Design review of the part built by this model. Coordinates are the model's own, in mm. Face numbers are marked on the shaded views. A direction names the side the tool comes from. Round coordinates to 2 decimals unless told otherwise and drop trailing zeros. Loops run counter-clockwise (first coordinate to the right, second up) from the corner with the lowest first, then second, coordinate; pieces in that order, holes last. Notation, with made-up numbers: (55, -4) - (106, -4) arc R29 cw to (106, 27) - close; hole circle Ø10 at (53, -17.5). An arc over 180 degrees is marked (long way). Use one line per item in the form item = value. Start each with the question number.
(1) We need section D-D, the plane x = 23.5. Write out the cut boundary in (y, z).
(2) For pin 1 (6 mm diameter, centred on x = 30.5, z = 15.5, fed in from -Y); pin 2 (3 mm diameter, centred on y = 4.5, z = 1.5, fed in from -X); pin 3 (3 mm diameter, centred on x = 52.5, z = 10.5, fed in from +Y), all flat-tipped, find the tip position at first contact; note any pin that passes through.
(3) Wall thickness on probe 1 along Z at (x, y) = (0, 3.5); probe 2 along Z at (x, y) = (31.95, -2.15); probe 3 along X at (y, z) = (5.1, 13.8): over which ranges is each line inside the solid? List them lowest first. Write a range as [from, to].
(4) The part is to be moulded in two halves that separate along Z. For the marked faces 1, 2, 3 and 4, say which applies: released by +Z, released by -Z, zero draft, split by the parting line, or undercut.
(5) We need section C-C, the plane z = -13.8. Write out the cut boundary in (x, y), then the cut area to 3 significant figures.
(6) We need section A-A, the plane x = 7.5. Write out the cut boundary in (y, z).
(7) Machinability: for the marked faces 5, 6, 7 and 8, which of the approach directions +Z, -Z, +X, -X, +Y, -Y give a long, thin tool a straight path to every point of the face, cutting with its end or side? Answer none if there is none.
(8) We need section B-B, the plane x = 55.95. Write out the cut boundary in (y, z).
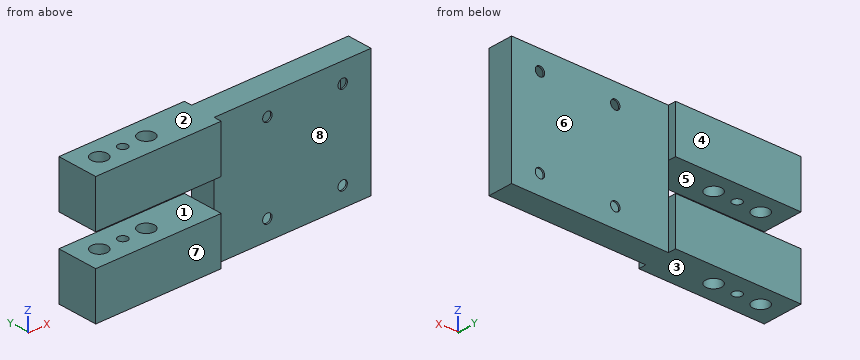
from build123d import *

# Parameters (mm, degrees)
BOSS_EXTRUDE1_DEPTH             = 5
BOSS_EXTRUDE1_DEPTH_BACK        = 5
SHELL1_T                        = -3
BOSS_EXTRUDE2_START             = 5
BOSS_EXTRUDE2_DEPTH             = 3
SKETCH2_R                       = 1.5
CUT_EXTRUDE1_DEPTH              = 100
SKETCH9_W                       = 40
SKETCH9_H                       = 2.5
CUT_EXTRUDE2_DEPTH              = 77.739820172
SKETCH10_W                      = 10
SKETCH10_H                      = 40
CUT_EXTRUDE3_DEPTH              = 2.5
CUT_EXTRUDE4_START              = -10.5
SKETCH10_2_W                    = 10
SKETCH10_2_H                    = 40
CUT_EXTRUDE4_DEPTH              = 2.5
F_3_0MM_CLEARANCE_DOWEL_HOLE1_D = 3
F_1_4_20_TAPPED_HOLE1_D         = 5.1054


with BuildPart() as part:
    # Sketch1 → Boss-Extrude1 (new, two sides: drawn at the far end of the back side and taken through both)
    with BuildSketch(Plane(origin=(0, 0, 0), x_dir=(1, 0, 0), z_dir=(0, 1, 0)).offset(-BOSS_EXTRUDE1_DEPTH_BACK)):
        Polygon((15, -5), (-25, -5), (-25, -20), (25, -20), (65, -20), (65, 20), (25, 20), (-25, 20), (-25, 5), (15, 5), align=None)
    extrude(amount=BOSS_EXTRUDE1_DEPTH + BOSS_EXTRUDE1_DEPTH_BACK)

    # Shell1
    shell1_openings = [part.faces().sort_by_distance(p)[0] for p in [
        (23.125, 5, 0),
    ]]
    offset(amount=SHELL1_T, openings=shell1_openings, kind=Kind.INTERSECTION)

    # Sketch1<2> → Boss-Extrude2 (add)
    with BuildSketch(Plane(origin=(0, 0, 0), x_dir=(1, 0, 0), z_dir=(0, 1, 0)).offset(BOSS_EXTRUDE2_START)):
        Polygon((15, -5), (-25, -5), (-25, -20), (25, -20), (65, -20), (65, 20), (25, 20), (-25, 20), (-25, 5), (15, 5), align=None)
    extrude(amount=BOSS_EXTRUDE2_DEPTH)

    # Sketch2 → Cut-Extrude1 (cut)
    with BuildSketch(Plane.XY.offset(20)):
        with Locations((-10.5, 1.5)):
            Circle(SKETCH2_R)
    extrude(amount=-CUT_EXTRUDE1_DEPTH, mode=Mode.SUBTRACT)

    # Sketch9 → Cut-Extrude2 (cut, through all)
    with BuildSketch(Plane.XY.offset(20)):
        with Locations((45, 6.75)):
            Rectangle(SKETCH9_W, SKETCH9_H)
        with Locations((45, -3.75)):
            Rectangle(SKETCH9_W, SKETCH9_H)
    extrude(amount=-CUT_EXTRUDE2_DEPTH, mode=Mode.SUBTRACT)

    # Sketch10 → Cut-Extrude3 (cut)
    with BuildSketch(Plane(origin=(0, 8, 0), x_dir=(1, 0, 0), z_dir=(0, 1, 0))):
        with Locations((20, 0)):
            Rectangle(SKETCH10_W, SKETCH10_H)
    extrude(amount=-CUT_EXTRUDE3_DEPTH, mode=Mode.SUBTRACT)

    # Sketch10<2> → Cut-Extrude4 (cut)
    with BuildSketch(Plane(origin=(0, 8, 0), x_dir=(1, 0, 0), z_dir=(0, 1, 0)).offset(CUT_EXTRUDE4_START)):
        with Locations((20, 0)):
            Rectangle(SKETCH10_2_W, SKETCH10_2_H)
    extrude(amount=-CUT_EXTRUDE4_DEPTH, mode=Mode.SUBTRACT)

    # Ø3.0mm Clearance Dowel Hole1 (through all)
    with Locations(Plane(origin=(0, 5.5, 0), x_dir=(1, 0, 0), z_dir=(0, 1, 0))):
        with Locations((31.950000364, 13.8), (31.950000364, -13.8), (55.950000364, -13.8), (55.950000364, 13.8)):
            Hole(F_3_0MM_CLEARANCE_DOWEL_HOLE1_D / 2)

    # 1/4-20 Tapped Hole1 (through all)
    with Locations(Plane.XY.offset(20)):
        with Locations((-18, 1.5), (-3, 1.5)):
            Hole(F_1_4_20_TAPPED_HOLE1_D / 2)


solid = part.part
Data:
q1.outline = (-2.5, -20) - (5.5, -20) - (5.5, 20) - (-2.5, 20) - close; hole (-2, -17) - (5, -17) - (5, 17) - (-2, 17) - close
q2.pin_1 = -2.5
q2.pin_2 = 15
q2.pin_3 = 5.5
q3.probe_1 = [-20, -17], [-8, -5], [5, 8], [17, 20]
q3.probe_2 = [-20, -15.3], [-12.3, 12.3], [15.3, 20]
q3.probe_3 = [-25, 30.45], [33.45, 54.45], [57.45, 65]
q4.face_1 = undercut
q4.face_2 = released by +Z
q4.face_3 = released by -Z
q4.face_4 = zero draft
q5.outline = (-25, -5) - (15, -5) - (15, -2.5) - (30.45, -2.5) - (30.45, -2) - (-22, -2) - (-22, 5) - (30.45, 5) - (30.45, 5.5) - (15, 5.5) - (15, 8) - (-25, 8) - close; (33.45, -2.5) - (54.45, -2.5) - (54.45, -2) - (33.45, -2) - close; (33.45, 5) - (54.45, 5) - (54.45, 5.5) - (33.45, 5.5) - close; (57.45, -2.5) - (65, -2.5) - (65, 5.5) - (57.45, 5.5) - (57.45, 5) - (62, 5) - (62, -2) - (57.45, -2) - close
q5.area = 326 mm^2
q6.outline = (-5, -20) - (8, -20) - (8, -5) - (-5, -5) - close; (-5, 5) - (8, 5) - (8, 20) - (-5, 20) - close; hole (-2, -17) - (5, -17) - (5, -8) - (-2, -8) - close; hole (-2, 8) - (5, 8) - (5, 17) - (-2, 17) - close
q7.face_5 = -X, +Y, -Y
q7.face_6 = +Z, -Z, +X, +Y
q7.face_7 = +Z, -Z, +X, -X, -Y
q7.face_8 = +Z, -Z, +X, -Y
q8.outline = (-2.5, -20) - (5.5, -20) - (5.5, -15.3) - (5, -15.3) - (5, -17) - (-2, -17) - (-2, -15.3) - (-2.5, -15.3) - close; (-2.5, -12.3) - (-2, -12.3) - (-2, 12.3) - (-2.5, 12.3) - close; (-2.5, 15.3) - (-2, 15.3) - (-2, 17) - (5, 17) - (5, 15.3) - (5.5, 15.3) - (5.5, 20) - (-2.5, 20) - close; (5, -12.3) - (5.5, -12.3) - (5.5, 12.3) - (5, 12.3) - close
